Can you work these out from the model? Positions are in its coordinate system, mm. Face numbers are marked on the shaded views. A direction names the side the tool comes from. Coordinates: 2 decimals unless noted, no trailing zeros. Order: outer loops, then holes, each group sorted by start corner. A loop starts at its lowest first (then second) coordinate and runs counter-clockwise, first axis right, second up. Notation, with made-up numbers: (33, 28) -> (56, 28) arc R14 cw to (56, 42) -> close; hole circle Ø5 at (77, -23.5). An arc over 180 degrees is marked (long way). Write item = value, one per line. Start each with the question number.
Autodesk Inventor part; units mm, degrees
ref_plane "YZ Plane" through (0, 0, 0) normal (1, 0, 0) x (0, 1, 0)
ref_plane "XZ Plane" through (0, 0, 0) normal (0, 1, 0) x (-1, 0, 0)
ref_plane "XY Plane" through (0, 0, 0) normal (0, 0, 1) x (1, 0, 0)
sketch "Sketch1" plane through (0, 0, 0) normal (0, 0, 1) x (1, 0, 0)
  line L0 (0, -22.5) -> (560, -22.5)
  line L1 (560, -22.5) -> (560, 22.5)
  line L2 (560, 22.5) -> (0, 22.5)
  line L3 (0, 22.5) -> (0, -22.5)
  line L4 (0, -22.5) -> (560, 22.5) construction
  line L5 (560, -22.5) -> (0, 22.5) construction
  point P0 (0, 0)
  point P1 (0, 0)
  dimension "d154" = 560
  dimension "d155" = 45
extrude "Plate3" add sketch "Sketch1" along normal blind 3
sketch "Sketch7" plane through (0, 19.5, 0) normal (0, 1, 0) x (-1, 0, 0)
  line L0 (-560, 0) -> (0, 0)
  line L1 (0, 0) -> (0, 105)
  line L2 (0, 105) -> (-560, 105)
  line L3 (-560, 105) -> (-560, 0)
edge flange "Flange3" height 105 angle 90 thickness 3 bend radius 5 thickness toward (0, 1, 0) relief round relief width 3 relief depth 1.5 edges at (280, 22.5, 3) wall of the first edge with corners at (560, 19.5, 0) (0, 19.5, 0) (0, 19.5, 105) (560, 19.5, 105)
bend "Bend3"
corner "Corner3"
sketch "Sketch11" plane through (0, 19.5, 105) normal (0, -1, 0) x (1, 0, 0)
  line L0 (0, -97) -> (560, -97)
  line L1 (560, -97) -> (560, 0)
  line L2 (560, 0) -> (0, 0)
  line L3 (0, -97) -> (0, 0)
  line L4 (0, 0) -> (-24.0074, 0)
  line L5 (-24.0074, 0) -> (-49.4388, -102)
  line L6 (-49.4388, -102) -> (-1, -102)
  line L7 (-1, -102) -> (-1, -97)
  line L8 (-1, -97) -> (0, -97)
  line L9 (560, -102) -> (0, -102)
  line L10 (-1, -102) -> (-46.6039, -90.6297)
  point P0 (0, -105)
  dimension "d193" = 1
  dimension "d194" = 24.0074
  dimension "d195" = 14
  dimension "d203" = 47
extrude "Extrusion6" add sketch "Sketch11" against normal up to surface (3 mm away) contours L8 L7 L10 L5 L4 L3
sketch "Sketch12" plane through (560, 19.5, 8) normal (0, -1, 0) x (1, 0, 0)
  line L0 (-511.7125, 66.6075) -> (-545.6729, 75.0748)
  line L1 (-545.6729, 75.0748) -> (-554.1401, 41.1144)
  line L2 (-554.1401, 41.1144) -> (-520.1798, 32.6472)
  line L3 (-520.1798, 32.6472) -> (-511.7125, 66.6075)
  line L4 (-511.7125, 66.6075) -> (-554.1401, 41.1144) construction
  line L5 (-545.6729, 75.0748) -> (-520.1798, 32.6472) construction
  circle A0 centre (-541.3936, 19.9006) radius 5.05
  circle A1 centre (-492.9179, 69.6511) radius 5.05
  circle A2 centre (-560.8386, 86.5856) radius 5.05
  line L6 (-492.9179, 69.6511) -> (-560.8386, 86.5856) construction
  line L7 (-560.8386, 86.5856) -> (-541.3936, 19.9006) construction
  line L8 (-541.3936, 19.9006) -> (-492.9179, 69.6511) construction
  line L9 (-528.6927, 70.8411) -> (-541.3936, 19.9006) construction
  line L10 (-584.0074, 97) -> (-606.6039, 6.3703)
  point P0 (-560, -8)
  point P1 (-532.9263, 53.861)
  point P2 (-544.0023, 9.4376)
  dimension "d206" = 35
  dimension "d207" = 35
  dimension "d208" = 10.1
  dimension "d209" = 70
  dimension "d210" = 60
  dimension "d211" = 25
  dimension "d213" = 12
  dimension "d214" = 60
extrude "Cut1" cut sketch "Sketch12" against normal blind 3
pattern_linear "Rectangular Pattern5" count 4 spacing 160 along (1, 0, 0) of "Cut1"
properties part number "DS-B-102 ridge bottom" material "Stainless Steel"
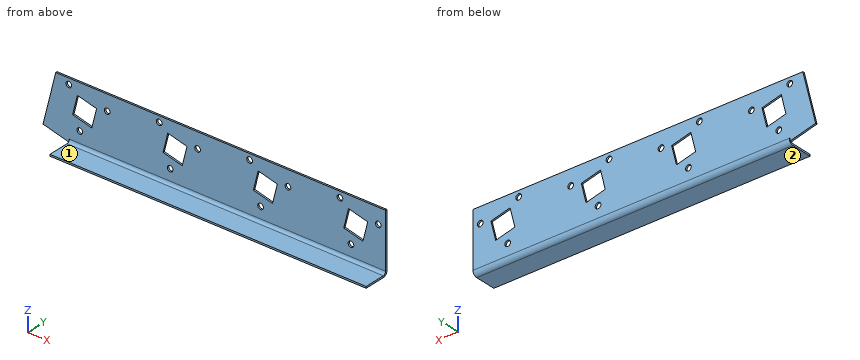
(1) For P1, Ø4, axis at y = 8, z = 2, coming from the -X side; P2, Ø2, axis at x = 64, y = -11.5, coming from the -Z side; P3, Ø13, axis at x = -0.84, z = 94.59, coming from the -Y side; P4, Ø11, axis at x = 239.5, y = 2.5, coming from the +Z side, each with a flat end and sliding along its axis, tell me the tip position at first contact or that it passes through.
(2) Imagine slicing it at A-A (x = 107). Write out the boundary of the cut face in (y, z), plus the area to 3 significant figures.
(3) If I drill on L1, parallel to Z at x = 235, y = 5; L2, parallel to Y at x = 516.5, z = 31; L3, parallel to Z at x = 288.5, y = 17.5, over which ranges is the centre line in solid material (lowest first)? Write a range as from..to.
(4) Imagine slicing it at B-B (y = -14). Write out the boundary of the cut face in (x, z), plus the area to 3 significant figures.
(5) For the marked faces 1 and 2, which set-ups out of +Z, -Z, +X, -X, +Y, -Y let a thin tool reach every point of the face, with its end or its side?
Result set:
q1.P1 = 0
q1.P2 = 0
q1.P3 = 19.5
q1.P4 = 3
q2.outline = (-22.5, 0) -> (14.5, 0) arc R8 ccw to (22.5, 8) -> (22.5, 105) -> (19.5, 105) -> (19.5, 8) arc R5 cw to (14.5, 3) -> (-22.5, 3) -> close
q2.area = 433 mm2
q3.L1 = 0..3
q3.L2 = 19.5..22.5
q3.L3 = 0.58..4
q4.outline = (0, 0) -> (560, 0) -> (560, 3) -> (0, 3) -> close
q4.area = 1,680 mm2
q5.face_1 = +Z, +X, -X, -Y
q5.face_2 = -Z, +X, -X, +Y, -Y
